```python
from build123d import *

# Parameters (mm, degrees)
F0_W      = 38.1
F0_H      = 38.1
F1_DEPTH  = 38.1
F6_DEPTH  = 38.1
F8_DEPTH  = 38.1
F10_DEPTH = 38.1
F11_W     = 25.183282
F11_H     = 6.221752
F12_DEPTH = 38.1


with BuildPart() as f1:
    # F0 (on Front) → F1 (new body)
    with BuildSketch(Plane.XZ):
        with Locations((19.05, 19.05)):
            Rectangle(F0_W, F0_H)
    extrude(amount=F1_DEPTH)

    # F5 (on offset) → F6 (cut)
    with BuildSketch(Plane.YZ.offset(38.1)):
        Polygon((-6.35, 38.1), (-31.75, 38.1), (-26.67, 14.842794), (-21.59, 28.575), (-16.51, 28.575), (-11.43, 14.842794), align=None)
        Polygon((-38.1, 38.1), (-38.1, 0), (-31.75, 0), align=None)
        Polygon((-19.05, 16.785284), (-25.4, 0), (-12.7, 0), align=None)
        Polygon((0, 38.1), (-6.35, 0), (0, 0), align=None)
    extrude(amount=-F6_DEPTH, mode=Mode.SUBTRACT)

    # F7 (on offset) → F8 (cut)
    with BuildSketch(Plane.XZ.offset(38.1)):
        Polygon((25.4, 38.1), (12.7, 38.1), (19.05, 18.617285), align=None)
        Polygon((0, 38.1), (0, 0), (6.35, 38.1), align=None)
        Polygon((11.43, 18.617285), (6.35, 0), (31.75, 0), (26.67, 18.617285), (21.59, 7.313934), (16.51, 7.313934), align=None)
        Polygon((31.75, 38.1), (38.1, 0), (38.1, 38.1), align=None)
    extrude(amount=-F8_DEPTH, mode=Mode.SUBTRACT)

    # F9 (on offset) → F10 (cut)
    with BuildSketch(Plane.XY.offset(38.1)):
        Polygon((25.308223, -23.404286), (0, -22.86), (0, -30.48), (25.308223, -30.48), align=None)
    extrude(amount=-F10_DEPTH, mode=Mode.SUBTRACT)

    # F11 (on offset) → F12 (cut)
    with BuildSketch(Plane.XY.offset(38.1)):
        with Locations((25.390372, -9.81442)):
            Rectangle(F11_W, F11_H)
    extrude(amount=-F12_DEPTH, mode=Mode.SUBTRACT)


solid = f1.part
```
Model file for the job. Use its own axes, mm. A direction names the side the tool comes from. Give positions to 0.01 mm unless a question says otherwise; leave off trailing zeros. Write each loop counter-clockwise with the first axis right and the second up, starting at its lowest first coordinate (ties: lowest second). Pieces come first, ordered by that corner, then holes. Notation, with made-up numbers: (0, 10.5) -> (53, 10.5) arc R25 ccw to (53, 39.5) -> close; hole circle Ø7 at (-22.5, 72). An arc over 180 degrees is marked (long way). Use CSV: the item, a comma, the result in double quotes. Start each with the question number.
1) Cut at A-A on y = -36. List the corners of the cut face in (x, z).
2) Cut at D-D on x = 14. List the corners of the cut face in (y, z) (3 decimals), plus the area to 3 significant figures.
3) Tool access for faces 3 (the flat face through (28, -19, 28.575)), 4 (the flat face through (12, -30.48, 20)), 5 (the flat face through (22.18, -33.5, 28.22)): list every direction of +Z, -Z, +X, -X, +Y, -Y with a clear straight run to the whole face (end or side of a thin tool).
4) Drill centre lines: L1, parallel to Y at x = 26, z = 20.5; L2, parallel to Y at x = 9, z = 12; L3, parallel to Y at x = 6, z = 29. Where is each one in solid material? Low to high.
5) Pin check, flat tips, straight feed: P1, Ø1.5, axis at x = 8, y = -19.5, coming from the +Z side (3 decimals); P2, Ø0.6, axis at x = 19.5, y = -23, coming from the -Z side; P3, Ø2, axis at y = -19, z = 20.5, coming from the +X side. Stop position of each tip, or through.
6) Cut at C-C on z = 25.5. List the corners of the cut face in (x, y), plus the area to 3 significant figures.
7) Two-plate mould, pull along Y, no slides. Class faces 1 (the flat face through (22.18, -4.14, 28.22)), 2 (the flat face through (10.053, -31.124, 35.234)): released by +Y, released by -Y, zero draft, split by the parting line, or undercut.
8) Cut at B-B on x = 3.5. List the corners of the cut face in (y, z).
Final values:
1,outline,"(4.25, 25.5) -> (16.81, 25.5) -> (12.7, 38.1) -> (6.35, 38.1) -> close; (21.29, 25.5) -> (33.85, 25.5) -> (31.75, 38.1) -> (25.4, 38.1) -> close"
2,outline,"(-37.435, 34.111) -> (-33.9, 12.899) -> (-30.48, 12.899) -> (-30.48, 32.286) -> (-30.879, 34.111) -> close; (-23.161, 12.899) -> (-20.52, 12.899) -> (-19.05, 16.785) -> (-17.58, 12.899) -> (-12.925, 12.899) -> (-12.925, 18.885) -> (-16.51, 28.575) -> (-21.59, 28.575) -> (-23.161, 24.328) -> close; (-6.704, 12.899) -> (-4.2, 12.899) -> (-0.665, 34.111) -> (-6.704, 34.111) -> close"
2,area,"334 mm2"
3,face 3,"+Z, +X, -X"
3,face 4,"+Z, -Z, -X"
3,face 5,"+Z, +Y, -Y"
4,L1,"y = -35.17 to -27.91, -24.58 to -13.52, -6.7 to -2.93"
4,L2,"y = -33.75 to -30.48, -23.05 to -20.86, -17.24 to -4.35"
4,L3,"y = -36.58 to -30.48, -8.34 to -1.52"
5,P1,"stops at z = 28.575"
5,P2,"stops at z = 7.31"
5,P3,"stops at x = 34.85"
6,outline,"(4.25, -36) -> (16.81, -36) -> (16.81, -30.48) -> (4.25, -30.48) -> close; (4.25, -22.73) -> (16.81, -22.73) -> (16.81, -15.37) -> (4.25, -15.37) -> close; (4.25, -9.1) -> (12.8, -9.1) -> (12.8, -6.7) -> (16.81, -6.7) -> (16.81, -2.1) -> (4.25, -2.1) -> close; (21.29, -36) -> (33.85, -36) -> (33.85, -29) -> (25.31, -29) -> (25.31, -30.48) -> (21.29, -30.48) -> close; (21.29, -22.73) -> (33.85, -22.73) -> (33.85, -15.37) -> (21.29, -15.37) -> close; (21.29, -6.7) -> (33.85, -6.7) -> (33.85, -2.1) -> (21.29, -2.1) -> close"
6,area,"472 mm2"
7,face 1,"zero draft"
7,face 2,"undercut"
8,outline,"(-35.25, 21) -> (-31.75, 0) -> (-30.48, 0) -> (-30.48, 21) -> close; (-22.94, 6.52) -> (-19.05, 16.79) -> (-12.7, 0) -> (-6.35, 0) -> (-2.85, 21) -> (-10.09, 21) -> (-11.43, 14.84) -> (-13.71, 21) -> (-22.94, 21) -> close"
